For this review, take the finished solid that the model builds, in its own axes (mm). Face numbers are marked on the shaded views. A direction names the side the tool comes from. Coordinates: 2 decimals unless noted, no trailing zeros. Order: outer loops, then holes, each group sorted by start corner. A loop starts at its lowest first (then second) coordinate and runs counter-clockwise, first axis right, second up.
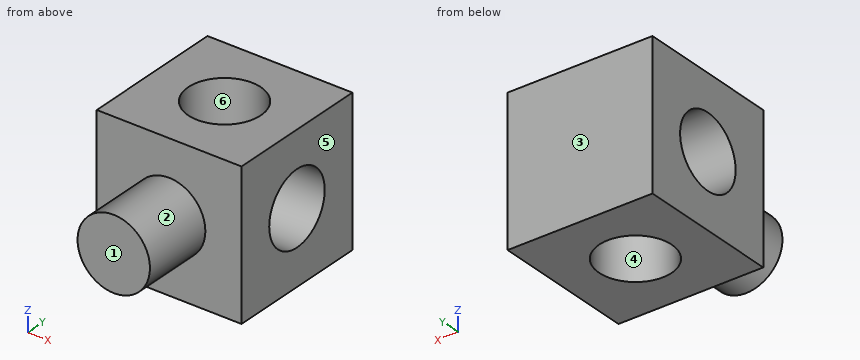
from build123d import *

# Parameters (mm, degrees)
F1_R     = 12.700524
F2_DEPTH = 25.4
F0_W     = 50.799996
F0_H     = 51.030912
F3_DEPTH = 50.8
F5_D     = 25.4508
F7_D     = 25.4508


with BuildPart() as f2:
    # F1 (on Front) → F2 (new body)
    with BuildSketch(Plane.XZ):
        Circle(F1_R)
    extrude(amount=F2_DEPTH)

    # F0 (on Front) → F3 (join)
    with BuildSketch(Plane.XZ):
        Rectangle(F0_W, F0_H)
    extrude(amount=-F3_DEPTH)

    # F5 (through all)
    with Locations(Plane.YZ.offset(25.399998)):
        with Locations((25.4, 0)):
            Hole(F5_D / 2)

    # F7 (through all)
    with Locations(Plane.XY.offset(25.515456)):
        with Locations((0, 25.4)):
            Hole(F7_D / 2)


solid = f2.part
1. Take a section at C-C, the plane z = -5.5. Give the boundary of the cut face in (x, y).
Answer below:
outline: (-25.4, 0) - (-11.45, 0) - (-11.45, -25.4) - (11.45, -25.4) - (11.45, 0) - (25.4, 0) - (25.4, 13.92) - (5.5, 13.92) arc R12.73 cw to (-5.5, 13.92) - (-25.4, 13.92) - close; (-25.4, 36.88) - (-5.5, 36.88) arc R12.73 cw to (5.5, 36.88) - (25.4, 36.88) - (25.4, 50.8) - (-25.4, 50.8) - close
2. To check wall thickness, follow L1, parallel to X at y = 25, z = 19; L2, parallel to Z at x = -17.25, y = 25.4; L3, parallel to Y at x = 7, z = 9.5. State the ranges of each line that lie inside material, in increasing order.
Answer below:
L1: x = -25.4 to -12.72, 12.72 to 25.4
L2: z = -25.52 to -12.73, 12.73 to 25.52
L3: y = -25.4 to 14.77, 36.03 to 50.8
3. The part is to be moulded in two halves that separate along Y. For the marked faces 3, 4, 5 and 6, say which applies: +Y half, -Y half, draft (parallel to the pull), parting line (faces both ways), or undercut.
Answer below:
face 3: +Y half
face 4: undercut
face 5: draft
face 6: undercut
4. Machinability: for the marked faces 1 and 2, which of the approach directions +Z, -Z, +X, -X, +Y, -Y give a long, thin tool a straight path to every point of the face, cutting with its end or side? Answer none if there is none.
Answer below:
face 1: +Z, -Z, +X, -X, -Y
face 2: -Y
5. Take a section at A-A, the plane y = 14.5. Give the boundary of the cut face in (x, z), plus the area to 3 significant figures.
Answer below:
outline: (-25.4, -25.52) - (-6.57, -25.52) - (-6.57, -6.57) - (-25.4, -6.57) - close; (-25.4, 6.57) - (-6.57, 6.57) - (-6.57, 25.52) - (-25.4, 25.52) - close; (6.57, -25.52) - (25.4, -25.52) - (25.4, -6.57) - (6.57, -6.57) - close; (6.57, 6.57) - (25.4, 6.57) - (25.4, 25.52) - (6.57, 25.52) - close
area: 1,430 mm2
6. Take a section at D-D, the plane z = 21.5. Give the boundary of the cut face in (x, y), plus the area to 3 significant figures.
Answer below:
outline: (-25.4, 0) - (25.4, 0) - (25.4, 50.8) - (-25.4, 50.8) - close; hole circle Ø25.45 at (0, 25.4)
area: 2,070 mm2
7. Take a section at B-B, the plane x = -3. Give the boundary of the cut face in (y, z).
Answer below:
outline: (-25.4, -12.34) - (0, -12.34) - (0, -25.52) - (13.03, -25.52) - (13.03, -3) arc R12.73 cw to (13.03, 3) - (13.03, 25.52) - (0, 25.52) - (0, 12.34) - (-25.4, 12.34) - close; (37.77, -25.52) - (50.8, -25.52) - (50.8, 25.52) - (37.77, 25.52) - (37.77, 3) arc R12.73 cw to (37.77, -3) - close
8. Clearance check with flat-ended pins moving along their axes: pin 1 Ø6 at (y, z) = (-6.5, 14.5) entering from -X; pin 2 Ø6 at (x, y) = (-12, 25) entering from -Z; pin 3 Ø20.5 at (x, y) = (0, 25.4) entering from +Z; pin 4 Ø5 at (x, y) = (-7, -5) entering from +Z. State where each tip first meets the part, or that it passes through.
Answer below:
pin 1: stops at x = -5.39
pin 2: stops at z = -25.52
pin 3: passes through
pin 4: stops at z = 11.88
